Can you work these out from the model? Positions are in its coordinate system, mm. Face numbers are marked on the shaded views. A direction names the side the tool comes from. Coordinates: 2 decimals unless noted, no trailing zeros. Order: outer loops, then holes, each group sorted by start corner. A loop starts at its lowest first (then second) coordinate and runs counter-clockwise, first axis right, second up. Notation, with made-up numbers: (33, 64.5) - (39, 64.5) arc R20 ccw to (39, 81.5) - close; hole circle Ø6 at (14.5, 71). An arc over 180 degrees is marked (long way). Use a Markdown table: item, result. Add a question column.
(1) I want a section at B-B (z = -29). List the corners of the cut face in (x, y) for me, and give its area (3 significant figures).
(2) I want a section at C-C (x = -725.5). List the corners of the cut face in (y, z) for me.
(3) If I drill on L1, parallel to X at y = -11.5, z = -20; L2, parallel to X at y = 1, z = -9; L3, parallel to Z at x = -724, y = 11.5, over which ranges is the centre line in solid material (lowest first)? Write a range as [from, to].
(4) For pin 1 Ø6.5 at (x, y) = (-746, -10) entering from +Z; pin 2 Ø2 at (x, z) = (-731, -4.5) entering from +Y; pin 3 Ø4.5 at (y, z) = (-4.5, -13) entering from +X, each with a flat end and sliding along its axis, tell me the tip position at first contact or that it passes through.
(5) On a 3-axis mill with a long thin cutter (end or side, diameter ignored), from which of +Z, -Z, +X, -X, +Y, -Y can I reach the whole of each face in a straight line? I mean the marked faces 1, 2 and 3. Say none if no direction works.
(6) I want a section at D-D (y = -2.25). List the corners of the cut face in (x, z) for me, and give its area (3 significant figures).
(7) I want a section at A-A (z = -20). List the corners of the cut face in (x, y) for me.
(8) We'd pull the mould along Y, two halves only. Please class the marked faces 4, 5, 6 and 7: pulls with the +Y half, pulls with the -Y half, needs draft (parallel to the pull), parting line crosses it, or undercut.
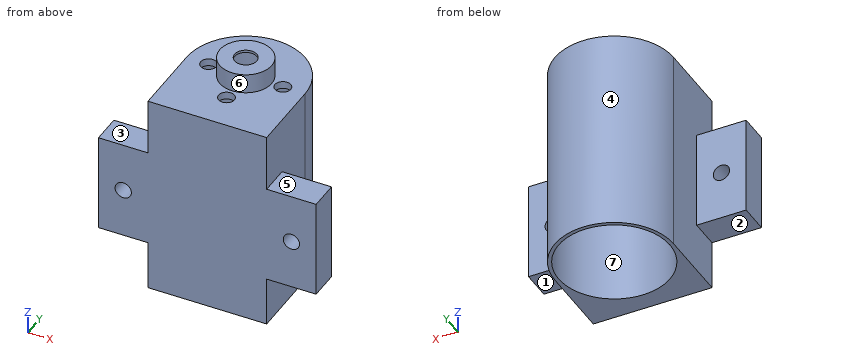
```python
from build123d import *
from build123d.topology import SkipClean

# Parameters (mm, degrees)
CROQUIS1_R              = 12
SALIENTE_EXTRUIR1_DEPTH = 1.5
CROQUIS2_R              = 1.606590309
CORTAR_EXTRUIR1_DEPTH   = 2
CROQUIS3_R              = 5.25
SALIENTE_EXTRUIR2_DEPTH = 4
CROQUIS4_R              = 5.1
CORTAR_EXTRUIR2_DEPTH   = 5
CROQUIS5_R              = 2.25
CORTAR_EXTRUIR3_DEPTH   = 5
SALIENTE_EXTRUIR3_START = 40
CROQUIS7_R              = 12
CROQUIS7_R_2            = 11.25
SALIENTE_EXTRUIR3_DEPTH = 40
SALIENTE_EXTRUIR4_DEPTH = 41.5
CROQUIS9_W              = 20
CROQUIS9_H              = 6
SALIENTE_EXTRUIR5_DEPTH = 10
CROQUIS10_W             = 20
CROQUIS10_H             = 6
SALIENTE_EXTRUIR6_DEPTH = 10
CROQUIS11_R             = 1.65
CORTAR_EXTRUIR4_DEPTH   = 10


with BuildPart() as part:
    # Croquis1 → Saliente-Extruir1 (new body)
    with BuildSketch(Plane.XY):
        with Locations((-728.422782565, 1.40916901)):
            Circle(CROQUIS1_R)
    extrude(amount=SALIENTE_EXTRUIR1_DEPTH)

    # Croquis2 → Cortar-Extruir1 (cut)
    with BuildSketch(Plane.XY.offset(1.5)):
        with Locations((-728.422782565, 8.90916901)):
            Circle(CROQUIS2_R)
        with Locations((-720.922782565, 1.40916901)):
            Circle(CROQUIS2_R)
        with Locations((-728.422782565, -6.09083099)):
            Circle(CROQUIS2_R)
        with Locations((-735.922782565, 1.40916901)):
            Circle(CROQUIS2_R)
    extrude(amount=-CORTAR_EXTRUIR1_DEPTH, mode=Mode.SUBTRACT)

    # Croquis3 → Saliente-Extruir2 (add)
    with BuildSketch(Plane.XY.offset(1.5)):
        with Locations((-728.422782565, 1.40916901)):
            Circle(CROQUIS3_R)
    extrude(amount=SALIENTE_EXTRUIR2_DEPTH)

    # Croquis4 → Cortar-Extruir2 (cut)
    with BuildSketch(Plane(origin=(0, 0, 0), x_dir=(-1, 0, 0), z_dir=(0, 0, -1))):
        with Locations((728.422782565, 1.40916901)):
            Circle(CROQUIS4_R)
    extrude(amount=-CORTAR_EXTRUIR2_DEPTH, mode=Mode.SUBTRACT)

    # Croquis5 → Cortar-Extruir3 (cut)
    with BuildSketch(Plane.XY.offset(5.5)):
        with Locations((-728.422782565, 1.40916901)):
            Circle(CROQUIS5_R)
    extrude(amount=-CORTAR_EXTRUIR3_DEPTH, mode=Mode.SUBTRACT)

    # Croquis7 → Saliente-Extruir3 (add)
    with BuildSketch(Plane(origin=(0, 0, 0), x_dir=(-1, 0, 0), z_dir=(0, 0, -1)).offset(SALIENTE_EXTRUIR3_START)):
        with Locations((728.422782565, 1.40916901)):
            Circle(CROQUIS7_R)
        with Locations((728.422782565, 1.40916901)):
            Circle(CROQUIS7_R_2, mode=Mode.SUBTRACT)
    extrude(amount=-SALIENTE_EXTRUIR3_DEPTH)

    # Croquis8 → Saliente-Extruir4 (add)
    with SkipClean():  # the faces are left unmerged after this step: merging them gives an invalid solid
        with BuildSketch(Plane(origin=(0, 0, -40), x_dir=(-1, 0, 0), z_dir=(0, 0, -1))):
            with BuildLine():
                Line((716.422782565, 1.40916901), (716.422782565, -13.59083099))
                Line((716.422782565, -13.59083099), (728.422782565, -13.59083099))
                Line((728.422782565, -13.59083099), (740.422782565, -13.59083099))
                Line((740.422782565, -13.59083099), (740.422782565, 1.40916901))
                ThreePointArc((740.422782565, 1.40916901), (728.422782565, -10.59083099), (716.422782565, 1.40916901))
            make_face()
        extrude(amount=-SALIENTE_EXTRUIR4_DEPTH)
    add(part.part.scale(1), mode=Mode.REPLACE)  # the faces are merged on a copy

    # Croquis9 → Saliente-Extruir5 (add)
    with BuildSketch(Plane.ZY.offset(740.422782565)):
        with Locations((-20, -10.59083099)):
            Rectangle(CROQUIS9_W, CROQUIS9_H)
    extrude(amount=SALIENTE_EXTRUIR5_DEPTH)

    # Croquis10 → Saliente-Extruir6 (add)
    with BuildSketch(Plane(origin=(-716.422782565, 0, 0), x_dir=(0, 0, -1), z_dir=(1, 0, 0))):
        with Locations((20, -10.59083099)):
            Rectangle(CROQUIS10_W, CROQUIS10_H)
    extrude(amount=SALIENTE_EXTRUIR6_DEPTH)

    # Croquis11 → Cortar-Extruir4 (cut)
    with BuildSketch(Plane(origin=(0, -7.59083099, 0), x_dir=(1, 0, 0), z_dir=(0, 1, 0))):
        with Locations(Location((-745.422782565, 20, 0), (0, 0, 270))):
            Circle(CROQUIS11_R)
        with Locations(Location((-711.422782565, 20, 0), (0, 0, 270))):
            Circle(CROQUIS11_R)
    extrude(amount=-CORTAR_EXTRUIR4_DEPTH, mode=Mode.SUBTRACT)


solid = part.part
```
Answers follow:
| question | item | result |
|---|---|---|
| 1 | outline | (-750.42, -13.59) - (-706.42, -13.59) - (-706.42, -7.59) - (-716.42, -7.59) - (-716.42, 1.41) arc R12 ccw to (-740.42, 1.41) - (-740.42, -7.59) - (-750.42, -7.59) - close; hole circle Ø22.5 at (-728.42, 1.41) |
| 1 | area | 309 mm² |
| 2 | outline | (-13.59, -40) - (-9.45, -40) - (-9.45, 0) - (-2.77, 0) - (-2.77, 5) - (5.59, 5) - (5.59, 0) - (12.27, 0) - (12.27, -40) - (13.05, -40) - (13.05, 1.5) - (5.77, 1.5) - (5.77, 5.5) - (-2.95, 5.5) - (-2.95, 1.5) - (-13.59, 1.5) - close |
| 3 | L1 | x = [-750.42, -747.07], [-743.77, -713.07], [-709.77, -706.42] |
| 3 | L2 | x = [-740.42, -739.67], [-717.18, -716.42] |
| 3 | L3 | z = [0, 1.5] |
| 4 | pin 1 | stops at z = -10 |
| 4 | pin 2 | stops at y = 13.31 |
| 4 | pin 3 | stops at x = -716.42 |
| 5 | face 1 | -Z, +X, +Y, -Y |
| 5 | face 2 | -Z, -X, +Y, -Y |
| 5 | face 3 | +Z, -X, +Y, -Y |
| 6 | outline | (-740.42, -40) - (-739.06, -40) - (-739.06, 0) - (-731.98, 0) - (-731.98, 5) - (-724.87, 5) - (-724.87, 0) - (-717.78, 0) - (-717.78, -40) - (-716.42, -40) - (-716.42, 1.5) - (-724.66, 1.5) - (-724.66, 5.5) - (-732.19, 5.5) - (-732.19, 1.5) - (-740.42, 1.5) - close |
| 6 | area | 140 mm² |
| 7 | outline | (-750.42, -13.59) - (-747.07, -13.59) - (-747.07, -7.59) - (-750.42, -7.59) - close; (-743.77, -13.59) - (-713.07, -13.59) - (-713.07, -7.59) - (-716.42, -7.59) - (-716.42, 1.41) arc R12 ccw to (-740.42, 1.41) - (-740.42, -7.59) - (-743.77, -7.59) - close; (-709.77, -13.59) - (-706.42, -13.59) - (-706.42, -7.59) - (-709.77, -7.59) - close; hole circle Ø22.5 at (-728.42, 1.41) |
| 8 | face 4 | pulls with the +Y half |
| 8 | face 5 | needs draft |
| 8 | face 6 | parting line crosses it |
| 8 | face 7 | undercut |
